Check sheet for the modelled part. Datum: model origin and axes. Units: mm. Face numbers are marked on the shaded views. A direction names the side the tool comes from. Give positions to 0.01 mm unless a question says otherwise; leave off trailing zeros. Order: outer loops, then holes, each group sorted by start corner. A loop starts at its lowest first (then second) coordinate and runs counter-clockwise, first axis right, second up. Notation, with made-up numbers: (38.25, 83.25) -> (77.25, 83.25) arc R23 cw to (77.25, 119.25) -> close; hole circle Ø11 at (-17, 85.25). An arc over 180 degrees is marked (long way). Answer in a Markdown table with one row per item. Add a question column.
(1) Cross-section at A-A (y = 1.7). Record the cut outline in (x, z).
(2) Set-up check for the marked faces 4, 5 and 6: record each of +Z, -Z, +X, -X, +Y, -Y from which the full face is reachable in a straight line by a thin tool's end or side.
(3) Thickness scan on L1, parallel to Z at x = 2.25, y = 1.75; L2, parallel to Y at x = 6.75, z = -3.25; L3, parallel to Y at x = 6, z = -3.75. Record the ranges inside material, lowest first. Write a range as [from, to].
(4) Go/stop test with a flat-tipped pin: pin 1 (3 mm diameter, centred on x = 3, z = -2, fed in from -Y). Record where the tip stops, or that it passes through.
(5) Cross-section at B-B (x = 4). Record the cut outline in (y, z), then the cut area to 3 significant figures.
(6) Cross-section at C-C (z = -4). Record the cut outline in (x, y), then the cut area to 3 significant figures.
(7) Release check for a two-part mould opening along Z. For the marked faces 1, 2 and 3 record: released by +Z, released by -Z, zero draft, split by the parting line, or undercut.
```python
from build123d import *

# Parameters (mm, degrees)
SKETCH1_W           = 8
SKETCH1_H           = 8
BOSS_EXTRUDE1_DEPTH = 3.2
SKETCH2_R           = 2.4
BOSS_EXTRUDE2_DEPTH = 1.8
SKETCH3_W           = 4.8
SKETCH3_H           = 4.8
CUT_EXTRUDE1_DEPTH  = 1.8


with BuildPart() as part:
    # Sketch1 → Boss-Extrude1 (new body)
    with BuildSketch(Plane(origin=(0, 0, 0), x_dir=(1, 0, 0), z_dir=(0, 1, 0))):
        with Locations((4, 4)):
            Rectangle(SKETCH1_W, SKETCH1_H)
    extrude(amount=BOSS_EXTRUDE1_DEPTH)

    # Sketch2 → Boss-Extrude2 (add)
    with BuildSketch(Plane(origin=(0, 3.2, 0), x_dir=(1, 0, 0), z_dir=(0, 1, 0))):
        with Locations(Location((4, 4, 0), (0, 0, 270))):
            Circle(SKETCH2_R)
    extrude(amount=BOSS_EXTRUDE2_DEPTH)

    # Sketch3 → Cut-Extrude1 (cut)
    with BuildSketch(Plane.XZ):
        with Locations((4, -4)):
            Rectangle(SKETCH3_W, SKETCH3_H)
    extrude(amount=-CUT_EXTRUDE1_DEPTH, mode=Mode.SUBTRACT)


solid = part.part
```
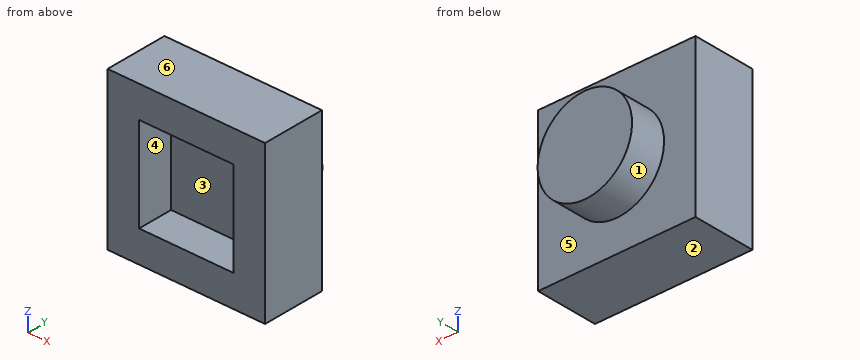
Answer below:
| question | item | result |
|---|---|---|
| 1 | outline | (0, -8) -> (8, -8) -> (8, 0) -> (0, 0) -> close; hole (1.6, -6.4) -> (6.4, -6.4) -> (6.4, -1.6) -> (1.6, -1.6) -> close |
| 2 | face 4 | -Y |
| 2 | face 5 | +Y |
| 2 | face 6 | +Z, +X, -X, +Y, -Y |
| 3 | L1 | z = [-8, -6.4], [-1.6, 0] |
| 3 | L2 | y = [0, 3.2] |
| 3 | L3 | y = [1.8, 5] |
| 4 | pin 1 | stops at y = 0 |
| 5 | outline | (0, -8) -> (3.2, -8) -> (3.2, -6.4) -> (5, -6.4) -> (5, -1.6) -> (3.2, -1.6) -> (3.2, 0) -> (0, 0) -> (0, -1.6) -> (1.8, -1.6) -> (1.8, -6.4) -> (0, -6.4) -> close |
| 5 | area | 25.6 mm² |
| 6 | outline | (0, 0) -> (1.6, 0) -> (1.6, 1.8) -> (6.4, 1.8) -> (6.4, 0) -> (8, 0) -> (8, 3.2) -> (6.4, 3.2) -> (6.4, 5) -> (1.6, 5) -> (1.6, 3.2) -> (0, 3.2) -> close |
| 6 | area | 25.6 mm² |
| 7 | face 1 | split by the parting line |
| 7 | face 2 | released by -Z |
| 7 | face 3 | undercut |
